```python
from build123d import *

# Parameters (mm, degrees)
SKETCH_2_R          = 1.5
EXTRUDE_1_DEPTH     = 7
CUT_EXTRUDE_1_DEPTH = 5
SKETCH_4_R          = 1.5
EXTRUDE_2_DEPTH     = 1


with BuildPart() as part:
    # 草图2 → 凸台-拉伸1 (new body)
    with BuildSketch(Plane(origin=(0, 0, 0), x_dir=(0, 0, -1), z_dir=(1, 0, 0))):
        with BuildLine():
            Line((0, 4), (37, 4))
            ThreePointArc((37, 4), (41, 0), (37, -4))
            Line((37, -4), (0, -4))
            ThreePointArc((0, -4), (-4, 0), (0, 4))
        make_face()
        Circle(SKETCH_2_R, mode=Mode.SUBTRACT)
        with Locations((37, 0)):
            Circle(SKETCH_2_R, mode=Mode.SUBTRACT)
    extrude(amount=EXTRUDE_1_DEPTH)

    # 草图3 → 切除-拉伸1 (cut)
    with BuildSketch(Plane(origin=(7, 0, 0), x_dir=(0, 0, -1), z_dir=(1, 0, 0))):
        with BuildLine():
            Line((15.5, -2), (6, -2))
            ThreePointArc((6, -2), (4, 0), (6, 2))
            Line((6, 2), (15.5, 2))
            ThreePointArc((15.5, 2), (17.5, 0), (15.5, -2))
        make_face()
        with BuildLine():
            Line((21.5, -2), (31, -2))
            ThreePointArc((31, -2), (33, 0), (31, 2))
            Line((31, 2), (21.5, 2))
            ThreePointArc((21.5, 2), (19.5, 0), (21.5, -2))
        make_face()
    extrude(amount=-CUT_EXTRUDE_1_DEPTH, mode=Mode.SUBTRACT)

    # 草图4 → 凸台-拉伸2 (add)
    # profile 1 of 2: a face of its own
    with BuildSketch(Plane(origin=(7, 0, 0), x_dir=(0, 0, -1), z_dir=(1, 0, 0))):
        with BuildLine():
            ThreePointArc((37, -4), (39.828427125, -2.828427125), (41, 0))
            ThreePointArc((41, 0), (39.828427125, 2.828427125), (37, 4))
            ThreePointArc((37, 4), (33, 0), (37, -4))
        make_face()
        with Locations((37, 0)):
            Circle(SKETCH_4_R, mode=Mode.SUBTRACT)
    # profile 2 of 2: a face of its own
    with BuildSketch(Plane(origin=(7, 0, 0), x_dir=(0, 0, -1), z_dir=(1, 0, 0))):
        with BuildLine():
            ThreePointArc((0, -4), (2.828427125, -2.828427125), (4, 0))
            ThreePointArc((4, 0), (2.828427125, 2.828427125), (0, 4))
            ThreePointArc((0, 4), (-4, 0), (0, -4))
        make_face()
        Circle(SKETCH_4_R, mode=Mode.SUBTRACT)
    extrude(amount=EXTRUDE_2_DEPTH)


solid = part.part
```
Geometry: final body of the model. Coordinates: model frame, mm. A direction names the side the tool comes from. Coordinates: 2 decimals unless noted, no trailing zeros. Write each loop counter-clockwise with the first axis right and the second up, starting at its lowest first coordinate (ties: lowest second). Pieces come first, ordered by that corner, then holes. Notation, with made-up numbers: M 1.25,1 L 26.25,1 A30 cw 26.25,23 Z; hole C 74.25,-2.5 d7. An arc over 180 degrees is marked long. Answer as CSV lines item,"result". Start each with the question number.
Q1. Cut plane C-C on z = -12.5. Return the cut outline in (x, y).
Q2. Mould query, pull axis Z, two halves, no side actions, for faces 1 (the flat face through (2, 0, -11)), 2 (the cylindrical face through (4.5, 0, -19.5)), 3 (the flat face through (0, 0, -19)). Classes: released by +Z, released by -Z, zero draft, split by the parting line, or undercut.
Q3. Cut plane A-A on x = 7.5. Return the cut outline in (y, z).
Q4. Line query: line 1 (Y direction, x = 2.75, z = -24); line 2 (Z direction, x = 4, y = -0.5); line 3 (Y direction, x = 3.25, z = -37). Output: solid intervals per line, ascending. Write a range as from..to.
Q5. Pin query (flat end, axial travel): P1, Ø4, axis at y = -0.5, z = -11, coming from the +X side; P2, Ø1.2, axis at y = 0.5, z = -13.5, coming from the +X side. Return the tip coordinate at first contact, or that it passes through.
Q6. Cut plane D-D on y = 1. Return the cut outline in (x, z), then the cut area to 3 significant figures.
Q7. Cut plane B-B on x = 3. Return the cut outline in (y, z), then the cut area to 3 significant figures.
Q8. Reachability of faces 4 (the flat face through (8, 0, -2)), 5 (the flat face through (5, 2, -26)) from +Z, -Z, +X, -X, +Y, -Y: full face, straight path, thin tool, end or side. Return the list, or none.
Findings below:
1,outline,"M 0,-4 L 7,-4 L 7,-2 L 2,-2 L 2,2 L 7,2 L 7,4 L 0,4 Z"
2,face 1,"undercut"
2,face 2,"undercut"
2,face 3,"zero draft"
3,outline,"C 0,-37 d8; C 0,0 d8; hole C 0,-37 d3; hole C 0,0 d3"
4,line 1,"y = -4..-2, 2..4"
4,line 2,"z = -40.97..-38.41, -35.59..-32.94, -19.56..-17.44, -4.06..-1.41, 1.41..3.97"
4,line 3,"y = -4..-1.5, 1.5..4"
5,P1,"stops at x = 7"
5,P2,"stops at x = 2"
6,outline,"M 0,-40.87 L 8,-40.87 L 8,-38.12 L 0,-38.12 Z; M 0,-35.88 L 8,-35.88 L 8,-33.13 L 7,-33.13 L 7,-32.73 L 2,-32.73 L 2,-19.77 L 7,-19.77 L 7,-17.23 L 2,-17.23 L 2,-4.27 L 7,-4.27 L 7,-3.87 L 8,-3.87 L 8,-1.12 L 0,-1.12 Z; M 0,1.12 L 8,1.12 L 8,3.87 L 0,3.87 Z"
6,area,"163 mm2"
7,outline,"M -4,-37 A4 ccw 4,-37 L 4,0 A4 ccw -4,0 Z; hole M -2,-31 A2 ccw 2,-31 L 2,-21.5 A2 ccw -2,-21.5 Z; hole M -2,-15.5 A2 ccw 2,-15.5 L 2,-6 A2 ccw -2,-6 Z; hole C 0,-37 d3; hole C 0,0 d3"
7,area,"231 mm2"
8,face 4,"+Z, -Z, +X, +Y, -Y"
8,face 5,"+X"
